Read the model definition and answer for the solid it produces. Units are mm, in the model's axes. A direction names the side the tool comes from. Coordinates: 2 decimals unless noted, no trailing zeros. Order: outer loops, then holes, each group sorted by start corner. A loop starts at its lowest first (then second) coordinate and runs counter-clockwise, first axis right, second up. Notation, with made-up numbers: (44.5, 42.5) -> (66.5, 42.5) arc R16 ccw to (66.5, 57.5) -> close; hole circle Ø11 at (61.25, -31.5). An arc over 180 degrees is marked (long way). Return JSON: item names as keys, results as strings. Group by question number.
```python
from build123d import *

# Parameters (mm, degrees)
F0_W     = 222.25
F0_H     = 101.6
F1_DEPTH = 9.525
F2_W     = 7.112
F2_H     = 38.1
F3_DEPTH = 9.526
F4_W     = 7.112
F4_H     = 31.75
F5_DEPTH = 3.175
F6_W     = 208.026
F6_H     = 3.175
F6_W_2   = 3.175
F6_H_2   = 50.8
F7_DEPTH = 3.175
F9_DEPTH = 6.35


with BuildPart() as f1:
    # F0 (on Top) → F1 (new body)
    with BuildSketch(Plane.XY):
        Rectangle(F0_W, F0_H)
    extrude(amount=F1_DEPTH)

    # F2 (on face) → F3 (cut, through all)
    with BuildSketch(Plane.XY.offset(9.525)):
        with Locations((-107.569, 0)):
            Rectangle(F2_W, F2_H)
        with Locations((107.569, 0)):
            Rectangle(F2_W, F2_H)
    extrude(amount=-F3_DEPTH, mode=Mode.SUBTRACT)

    # F4 (on face) → F5 (cut)
    with BuildSketch(Plane.XY.offset(9.525)):
        Polygon((-111.125, 19.05), (-104.013, 19.05), (-104.013, 46.0248), (104.013, 46.0248), (104.013, 19.05), (111.125, 19.05), (111.125, 50.8), (-111.125, 50.8), align=None)
        with Locations((-107.569, -34.925)):
            Rectangle(F4_W, F4_H)
        with Locations((107.569, -34.925)):
            Rectangle(F4_W, F4_H)
    extrude(amount=-F5_DEPTH, mode=Mode.SUBTRACT)

    # F6 (on face) → F7 (cut)
    with BuildSketch(Plane.XY.offset(9.525)):
        with Locations((0, -42.8625)):
            Rectangle(F6_W, F6_H)
        Polygon((-50.8, -4.7752), (-104.013, -4.7752), (-104.013, -7.9502), (104.013, -7.9502), (104.013, -4.7752), (-19.05, -4.7752), (-22.225, -4.7752), (-47.625, -4.7752), align=None)
        with Locations((-49.2125, 20.6248)):
            Rectangle(F6_W_2, F6_H_2)
        with Locations((-20.6375, 20.6248)):
            Rectangle(F6_W_2, F6_H_2)
    extrude(amount=-F7_DEPTH, mode=Mode.SUBTRACT)

    # F8 (on face) → F9 (cut, through all)
    with BuildSketch(Plane(origin=(0, 0, 0), x_dir=(1, 0, 0), z_dir=(0, 0, -1))):
        with BuildLine():
            Line((104.013, -19.05), (104.013, -18.415))
            ThreePointArc((104.013, -18.415), (103.563987, -19.499013), (104.648, -19.05))
            Line((104.648, -19.05), (104.013, -19.05))
        make_face()
        with BuildLine():
            ThreePointArc((104.648, 19.05), (103.563987, 19.499013), (104.013, 18.415))
            Line((104.013, 18.415), (104.013, 19.05))
            Line((104.013, 19.05), (104.648, 19.05))
        make_face()
        with BuildLine():
            Line((-104.013, 19.05), (-104.013, 18.415))
            ThreePointArc((-104.013, 18.415), (-103.563987, 19.499013), (-104.648, 19.05))
            Line((-104.648, 19.05), (-104.013, 19.05))
        make_face()
        with BuildLine():
            ThreePointArc((-104.648, -19.05), (-103.563987, -19.499013), (-104.013, -18.415))
            Line((-104.013, -18.415), (-104.013, -19.05))
            Line((-104.013, -19.05), (-104.648, -19.05))
        make_face()
    extrude(amount=-F9_DEPTH, mode=Mode.SUBTRACT)


solid = f1.part
```
1. Find section A-A on y = 31.5. Determine the outline of the cut face in (x, z) (3 decimals).
2. For a pull along Y with two mould halves and no side action, classify faces 1 (the face through (-2, -50.8, 5)), 2 (the face through (-1, -24, 9.525)), 3 (the face through (108, -19.05, 3)) as released by +Y, released by -Y, zero draft, split by the parting line, or undercut.
3. Given pin 1 (1.6 mm diameter, centred on y = 13.5, z = 8.5, fed in from +X); pin 2 (1.5 mm diameter, centred on x = -85, z = 8, fed in from +Y); pin 3 (3 mm diameter, centred on y = 6, z = 7, fed in from -X), each flat-ended and moving along its own axis, determine where each tip first touches the part or whether it passes through.
4. Straight lines are drawn through the part: L1, parallel to X at y = 2.5, z = 7 (3 decimals); L2, parallel to Y at x = 15.5, z = 8.5 (3 decimals); L3, parallel to X at y = 18, z = 5. For each, find the intervals that lie inside material, in ascending order.
5. Find section B-B on x = -89.5. Determine the outline of the cut face in (y, z) (3 decimals), and give its area (3 significant figures).
6. Find section D-D on y = -12.5. Determine the outline of the cut face in (x, z) (3 decimals).
7. Find section C-C on y = 3. Determine the outline of the cut face in (x, z) (3 decimals).
8. Which of the six approach directions +Z, -Z, +X, -X, +Y, -Y give full straight-line access (tool end or side, diameter ignored) to faces 4 (the face through (-104.013, 2, 6)), 5 (the face through (104.013, 2, 6)), 6 (the face through (-1, -48, 9.525)), 7 (the face through (-108, -19.05, 3))?
Result:
{
 "1": {"outline": "(-111.125, 0) -> (111.125, 0) -> (111.125, 6.35) -> (104.013, 6.35) -> (104.013, 9.525) -> (-19.05, 9.525) -> (-19.05, 6.35) -> (-22.225, 6.35) -> (-22.225, 9.525) -> (-47.625, 9.525) -> (-47.625, 6.35) -> (-50.8, 6.35) -> (-50.8, 9.525) -> (-104.013, 9.525) -> (-104.013, 6.35) -> (-111.125, 6.35) -> close"},
 "2": {"face 1": "released by -Y", "face 2": "zero draft", "face 3": "undercut"},
 "3": {"pin 1": "x = 104.01", "pin 2": "y = 46.02", "pin 3": "x = -104.01"},
 "4": {"L1": "-104.013 to -50.8, -47.625 to -22.225, -19.05 to 104.013", "L2": "-50.8 to -44.45, -41.275 to -7.95, -4.775 to 46.025", "L3": "-104.01 to 104.01"},
 "5": {"outline": "(-50.8, 0) -> (50.8, 0) -> (50.8, 6.35) -> (46.025, 6.35) -> (46.025, 9.525) -> (-4.775, 9.525) -> (-4.775, 6.35) -> (-7.95, 6.35) -> (-7.95, 9.525) -> (-41.275, 9.525) -> (-41.275, 6.35) -> (-44.45, 6.35) -> (-44.45, 9.525) -> (-50.8, 9.525) -> close", "area": "932 mm^2"},
 "6": {"outline": "(-104.013, 0) -> (104.013, 0) -> (104.013, 9.525) -> (-104.013, 9.525) -> close"},
 "7": {"outline": "(-104.013, 0) -> (104.013, 0) -> (104.013, 9.525) -> (-19.05, 9.525) -> (-19.05, 6.35) -> (-22.225, 6.35) -> (-22.225, 9.525) -> (-47.625, 9.525) -> (-47.625, 6.35) -> (-50.8, 6.35) -> (-50.8, 9.525) -> (-104.013, 9.525) -> close"},
 "8": {"face 4": "+Z, -X", "face 5": "+Z, +X", "face 6": "+Z, +X, -X, +Y, -Y", "face 7": "+Z, -Z, -X"}
}
